Geometry: final body of the model. Coordinates: model frame, mm. Give positions to 0.01 mm unless a question says otherwise; leave off trailing zeros. Loops run counter-clockwise (first coordinate to the right, second up) from the corner with the lowest first, then second, coordinate; pieces in that order, holes last. Notation, with made-up numbers: M 29,11.5 L 45,11.5 A15 ccw 45,26.5 Z; hole C 68.25,37 d5. An arc over 180 degrees is marked long. One line per question, with ' | ' between items. Start each with the question number.
from build123d import *

# Parameters (mm, degrees)
ESQUISSE1_R                  = 15
ESQUISSE1_R_2                = 10.5
BOSS_EXTRU_1_DEPTH           = 30
ENL_V_MAT_EXTRU_1_DEPTH      = 37.742346142
ENL_V_MAT_EXTRU_1_DEPTH_BACK = 37.742346142
ESQUISSE2_R                  = 1.95
ENL_V_MAT_EXTRU_2_DEPTH      = 37.742346305
ENL_V_MAT_EXTRU_2_DEPTH_BACK = 37.742346305
ESQUISSE3_R                  = 1.8
ENL_V_MAT_EXTRU_3_DEPTH      = 37.742346305
ENL_V_MAT_EXTRU_3_DEPTH_BACK = 37.742346305
ESQUISSE4_R                  = 2
ENL_V_MAT_EXTRU_4_DEPTH      = 37.742346305
ENL_V_MAT_EXTRU_4_DEPTH_BACK = 37.742346305
ESQUISSE5_R                  = 1.85
ENL_V_MAT_EXTRU_5_DEPTH      = 37.742346305
ENL_V_MAT_EXTRU_5_DEPTH_BACK = 37.742346305
ESQUISSE6_R                  = 1.95


with BuildPart() as part:
    # Esquisse1 → Boss.-Extru.1 (new body)
    with BuildSketch(Plane.XY):
        Circle(ESQUISSE1_R)
        Circle(ESQUISSE1_R_2, mode=Mode.SUBTRACT)
    extrude(amount=BOSS_EXTRU_1_DEPTH)

    # Esquisse2 → Enlèv. mat.-Extru.1 (cut, two sides: drawn at the far end of the back side and taken through both)
    with BuildSketch(Plane(origin=(0, 0, 0), x_dir=(1, 0, 0), z_dir=(0, 1, 0)).offset(-ENL_V_MAT_EXTRU_1_DEPTH_BACK)):
        with Locations(Location((0, -3.761693036, 0), (0, 0, 270))):
            Circle(ESQUISSE2_R)
    extrude(amount=ENL_V_MAT_EXTRU_1_DEPTH + ENL_V_MAT_EXTRU_1_DEPTH_BACK, mode=Mode.SUBTRACT)

    # Esquisse3 → Enlèv. mat.-Extru.2 (cut, two sides: drawn at the far end of the back side and taken through both)
    with BuildSketch(Plane(origin=(0, 0, 0), x_dir=(1, 0, 0), z_dir=(0, 1, 0)).offset(-ENL_V_MAT_EXTRU_2_DEPTH_BACK)):
        with Locations(Location((0, -11.751934404, 0), (0, 0, 270))):
            Circle(ESQUISSE3_R)
    extrude(amount=ENL_V_MAT_EXTRU_2_DEPTH + ENL_V_MAT_EXTRU_2_DEPTH_BACK, mode=Mode.SUBTRACT)

    # Esquisse4 → Enlèv. mat.-Extru.3 (cut, two sides: drawn at the far end of the back side and taken through both)
    with BuildSketch(Plane(origin=(0, 0, 0), x_dir=(1, 0, 0), z_dir=(0, 1, 0)).offset(-ENL_V_MAT_EXTRU_3_DEPTH_BACK)):
        with Locations(Location((0, -19.287446587, 0), (0, 0, 270))):
            Circle(ESQUISSE4_R)
    extrude(amount=ENL_V_MAT_EXTRU_3_DEPTH + ENL_V_MAT_EXTRU_3_DEPTH_BACK, mode=Mode.SUBTRACT)

    # Esquisse5 → Enlèv. mat.-Extru.4 (cut, two sides: drawn at the far end of the back side and taken through both)
    with BuildSketch(Plane(origin=(0, 0, 0), x_dir=(1, 0, 0), z_dir=(0, 1, 0)).offset(-ENL_V_MAT_EXTRU_4_DEPTH_BACK)):
        with Locations(Location((0, -27.017842707, 0), (0, 0, 270))):
            Circle(ESQUISSE5_R)
    extrude(amount=ENL_V_MAT_EXTRU_4_DEPTH + ENL_V_MAT_EXTRU_4_DEPTH_BACK, mode=Mode.SUBTRACT)

    # Esquisse6 → Enlèv. mat.-Extru.5 (cut, two sides: drawn at the far end of the back side and taken through both)
    with BuildSketch(Plane(origin=(0, 0, 0), x_dir=(0, 0, -1), z_dir=(1, 0, 0)).offset(-ENL_V_MAT_EXTRU_5_DEPTH_BACK)):
        with Locations((-5.320764522, 0)):
            Circle(ESQUISSE6_R)
    extrude(amount=ENL_V_MAT_EXTRU_5_DEPTH + ENL_V_MAT_EXTRU_5_DEPTH_BACK, mode=Mode.SUBTRACT)


solid = part.part
Q1. Draft query along X for faces 1 (the cylindrical face through (0.079, 12.641, 9.954)), 2 (the flat face through (3.1, 10.2, 30)), 3 (the cylindrical face through (13.856, -5.745, 14.79)). Return one class per face: released by +X, released by -X, zero draft, split by the parting line, or undercut.
Q2. Section C-C, the plane y = 0. Output: boundary loops of the cut face in (x, z), plus the area to 3 significant figures.
Q3. Material intervals for L1, parallel to Z at x = 0, y = -11; L2, parallel to Z at x = 11.5, y = 0; L3, parallel to Y at x = 0, z = 23, sorted ascending.
Q4. Section D-D, the plane y = 7.5. Output: boundary loops of the cut face in (x, z).
Q5. Contact query for flat-ended pins moving along their axis: pin 1 (1.5 mm diameter, centred on x = 6, z = 8, fed in from -Y); pin 2 (3 mm diameter, centred on x = 0, z = 11.75, fed in from -Y); pin 3 (5 mm diameter, centred on y = -12, z = 15.5, fed in from +X); pin 4 (1.5 mm diameter, centred on y = -3.5, z = 16.5, fed in from -X). Output: stop coordinate, or through.
Q6. Section B-B, the plane z = 4.5. Output: boundary loops of the cut face in (x, y).
Q7. Section A-A, the plane y = 12. Output: boundary loops of the cut face in (x, z).
Model answer:
1) face 1: undercut | face 2: zero draft | face 3: split by the parting line
2) outline: M -15,0 L -10.5,0 L -10.5,3.37 L -15,3.37 Z; M -15,7.27 L -10.5,7.27 L -10.5,30 L -15,30 Z; M 10.5,0 L 15,0 L 15,3.37 L 10.5,3.37 Z; M 10.5,7.27 L 15,7.27 L 15,30 L 10.5,30 Z | area: 235 mm^2
3) L1: z = 0 to 1.81, 5.71 to 9.95, 13.55 to 17.29, 21.29 to 25.17, 28.87 to 30 | L2: z = 0 to 3.37, 7.27 to 30 | L3: y = -15 to -10.5, 10.5 to 15
4) outline: M -12.99,0 L -7.35,0 L -7.35,30 L -12.99,30 Z; M 7.35,0 L 12.99,0 L 12.99,30 L 7.35,30 Z
5) pin 1: stops at y = -14.05 | pin 2: passes through | pin 3: stops at x = 11.61 | pin 4: stops at x = -14.75
6) outline: M -14.9,-1.77 A15 ccw -1.8,-14.89 L -1.8,-10.34 A10.5 cw -10.35,-1.77 Z; M -14.9,1.77 L -10.35,1.77 A10.5 cw -1.8,10.34 L -1.8,14.89 A15 ccw Z; M 1.8,-14.89 A15 ccw 14.9,-1.77 L 10.35,-1.77 A10.5 cw 1.8,-10.34 Z; M 1.8,10.34 A10.5 cw 10.35,1.77 L 14.9,1.77 A15 ccw 1.8,14.89 Z
7) outline: M -9,0 L 9,0 L 9,30 L -9,30 Z; hole C 0,19.29 d4; hole C 0,3.76 d3.9; hole C 0,27.02 d3.7; hole C 0,11.75 d3.6
